The listing builds one solid part. Answer for the finished solid, in the listing's coordinates (mm). A direction names the side the tool comes from. Give positions to 0.01 mm unless a question says otherwise; leave off trailing zeros. Loops run counter-clockwise (first coordinate to the right, second up) from the corner with the lowest first, then second, coordinate; pieces in that order, holes last.
Item 1: The mould has two halves that part along X. Classify faces 1 (the face through (41, 0.5, -9.3)), 2 (the face through (33.07, 0.49, -4.81)), 3 (the face through (43, 0.5, -4.6)), 4 (the face through (23.086, 0.493, -4.208)): pulls with the +X half, pulls with the -X half, needs draft (parallel to the pull), parting line crosses it, or undercut.
Item 2: Section A-A, the plane x = 18 is taken. Give the vertices of the cut face in (y, z), and give its area (3 significant figures).
Item 3: Section C-C, the plane y = -5.75 is taken. Give the vertices of the cut face in (x, z).
Item 4: Section D-D, the plane x = 34.5 is taken. Give the vertices of the cut face in (y, z), and give its area (3 significant figures).
Item 5: Each of these flat-tipped pins is pushed along its axis until it touches: pin 1 Ø5 at (x, y) = (18, -5) entering from -Z; pin 2 Ø5 at (x, z) = (31.48, -4.6) entering from -Y; pin 3 Ø5 at (x, y) = (20.5, -4.5) entering from +Z; pin 4 Ø0.8 at (y, z) = (0.5, -4) entering from +X. Where does it stop, or does it pass through?
Item 6: A tool of negligible diameter and unlimited length cuts with its end or side. For faces 5 (the face through (5.594, 0.493, -5.719)), 6 (the face through (25, -5, -35)), 7 (the face through (44.4, 0.5, -20.3)), from which of +Z, -Z, +X, -X, +Y, -Y can it reach the whole face along a straight path? Write none if from no direction.
Item 7: Consider line 1 along X through (y, z) = (0.3, -24.6); line 2 along X through (y, z) = (0.6, -4.6); line 3 along Y through (x, z) = (18, -35.6). Determine where each line is inside the solid, lowest interval first.
Item 8: Section B-B, the plane z = -4 is taken. Give the vertices of the cut face in (x, y).
from build123d import *

# Parameters (mm, degrees)
SKETCH_1_R          = 1.6
EXTRUDE_1_DEPTH     = 1
SKETCH_2_W          = 50
SKETCH_2_H          = 1
EXTRUDE_2_DEPTH     = 11
SKETCH_3_R          = 1.6
CUT_EXTRUDE_1_DEPTH = 10


with BuildPart() as part:
    # 草图1 → 凸台-拉伸1 (new body)
    with BuildSketch(Plane(origin=(0, 0, 0), x_dir=(1, 0, 0), z_dir=(0, 1, 0))):
        with BuildLine():
            Line((8, 0), (43, 0))
            Line((43, 0), (43, 9.3))
            Line((43, 9.3), (39, 9.3))
            ThreePointArc((39, 9.3), (33.5, 14.8), (39, 20.3))
            Line((39, 20.3), (50, 20.3))
            Line((50, 20.3), (50, 36))
            Line((50, 36), (0, 36))
            Line((0, 36), (0, 8))
            ThreePointArc((0, 8), (5.656854249, 5.656854249), (8, 0))
        make_face()
        with Locations(Location((8.5, 24.6, 0), (0, 0, 270))):
            Circle(SKETCH_1_R, mode=Mode.SUBTRACT)
        with Locations(Location((21.5, 4, 0), (0, 0, 270))):
            Circle(SKETCH_1_R, mode=Mode.SUBTRACT)
        with Locations(Location((34.5, 24.6, 0), (0, 0, 90))):
            Circle(SKETCH_1_R, mode=Mode.SUBTRACT)
        with Locations(Location((31.481983771, 4.6, 0), (0, 0, 270))):
            Circle(SKETCH_1_R, mode=Mode.SUBTRACT)
        with Locations(Location((11.518016229, 4.6, 0), (0, 0, 90))):
            Circle(SKETCH_1_R, mode=Mode.SUBTRACT)
    extrude(amount=EXTRUDE_1_DEPTH)

    # 草图2 → 凸台-拉伸2 (add)
    with BuildSketch(Plane(origin=(0, 1, 0), x_dir=(1, 0, 0), z_dir=(0, 1, 0))):
        with Locations((25, 35.5)):
            Rectangle(SKETCH_2_W, SKETCH_2_H)
    extrude(amount=-EXTRUDE_2_DEPTH)

    # 草图3 → 切除-拉伸1 (cut)
    with BuildSketch(Plane.XY.offset(-35)):
        with Locations((46, -5)):
            Circle(SKETCH_3_R)
        with Locations((18, -5)):
            Circle(SKETCH_3_R)
    extrude(amount=-CUT_EXTRUDE_1_DEPTH, mode=Mode.SUBTRACT)


solid = part.part
Worked answers:
1. face 1: needs draft
1. face 2: undercut
1. face 3: pulls with the +X half
1. face 4: undercut
2. outline: (-10, -36) - (-6.6, -36) - (-6.6, -35) - (-10, -35) - close; (-3.4, -36) - (1, -36) - (1, 0) - (0, 0) - (0, -35) - (-3.4, -35) - close
2. area: 42.8 mm2
3. outline: (0, -36) - (16.59, -36) - (16.59, -35) - (0, -35) - close; (19.41, -36) - (44.59, -36) - (44.59, -35) - (19.41, -35) - close; (47.41, -36) - (50, -36) - (50, -35) - (47.41, -35) - close
4. outline: (-10, -36) - (1, -36) - (1, -26.2) - (0, -26.2) - (0, -35) - (-10, -35) - close; (0, -23) - (1, -23) - (1, -17.96) - (0, -17.96) - close; (0, -11.64) - (1, -11.64) - (1, 0) - (0, 0) - close
4. area: 36.5 mm2
5. pin 1: stops at z = -36
5. pin 2: stops at y = 0
5. pin 3: stops at z = -35
5. pin 4: stops at x = 43
6. face 5: +Z, -X, +Y, -Y
6. face 6: +Z, +X, -X, -Y
6. face 7: +X, +Y, -Y
7. line 1: x = 0 to 6.9, 10.1 to 32.9, 36.1 to 50
7. line 2: x = 6.55 to 9.92, 13.12 to 20.02, 22.98 to 29.88, 33.08 to 43
7. line 3: y = -10 to -6.6, -3.4 to 1
8. outline: (6.93, 0) - (10.03, 0) - (10.03, 1) - (6.93, 1) - close; (13, 0) - (19.9, 0) - (19.9, 1) - (13, 1) - close; (23.1, 0) - (30, 0) - (30, 1) - (23.1, 1) - close; (32.97, 0) - (43, 0) - (43, 1) - (32.97, 1) - close
